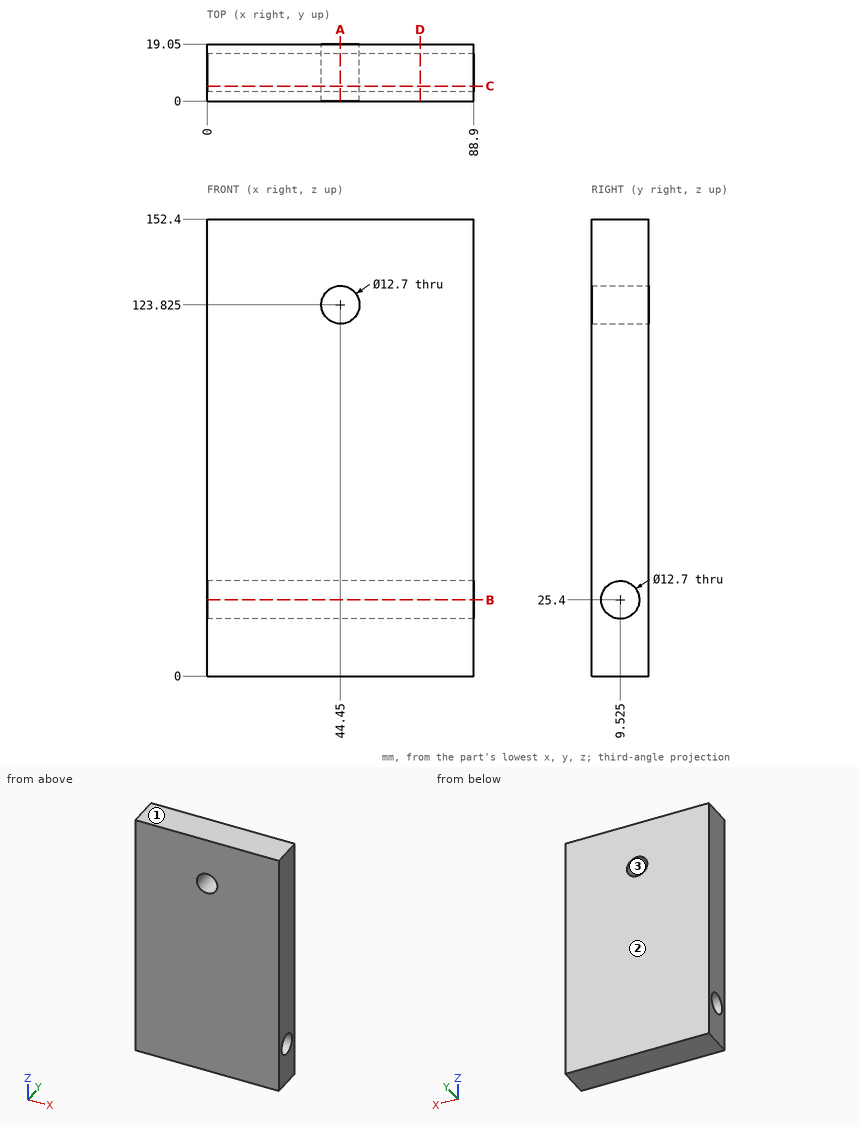
Study the drawing (mm; zero at the part's minimum x, y, z) and answer. Coordinates: 2 decimals unless noted, no trailing zeros. Write each loop counter-clockwise with the first axis right and the second up, starting at its lowest first coordinate (ties: lowest second). Pieces come first, ordered by that corner, then holes. Notation, with made-up numbers: (-15.75, 86.5) - (25.25, 86.5) arc R16 ccw to (25.25, 106.5) - close; hole circle Ø1 at (74.25, 82). An arc over 180 degrees is marked (long way). One line per item, written item: value.
1) Find section B-B (z = 25.4). Give the vertices of the cut face in (x, y) (3 decimals).
Geometry check:
outline: (0, 0) - (88.9, 0) - (88.9, 3.175) - (0, 3.175) - close; (0, 15.875) - (88.9, 15.875) - (88.9, 19.05) - (0, 19.05) - close
2) This flat-tipped pin is pushed along its axis until it touches: pin 1 Ø7.5 at (x, z) = (44.45, 123.825) entering from -Y. Where does it stop, or does it pass through?
Geometry check:
pin 1: passes through
3) Find section C-C (y = 5). Give the vertices of the cut face in (x, z) (3 decimals), and give its area (3 significant figures).
Geometry check:
outline: (0, 0) - (88.9, 0) - (88.9, 20.945) - (0, 20.945) - close; (0, 29.855) - (88.9, 29.855) - (88.9, 152.4) - (0, 152.4) - close; hole circle Ø12.7 at (44.45, 123.825)
area: 12,600 mm2
4) Find section A-A (x = 44.45). Give the vertices of the cut face in (y, z) (3 decimals), and give its area (3 significant figures).
Geometry check:
outline: (0, 0) - (19.05, 0) - (19.05, 117.475) - (0, 117.475) - close; (0, 130.175) - (19.05, 130.175) - (19.05, 152.4) - (0, 152.4) - close; hole circle Ø12.7 at (9.525, 25.4)
area: 2,530 mm2
5) Consider line 1 along Z through (x, y) = (15.5, 9); line 2 along Z through (x, y) = (40, 12.75); line 3 along Z through (x, y) = (43.5, 11.75). Determine where each line is inside the solid, lowest interval first. Write a range as from..to.
Geometry check:
line 1: z = 0..19.07, 31.73..152.4
line 2: z = 0..19.93, 30.87..119.3, 128.35..152.4
line 3: z = 0..19.45, 31.35..117.55, 130.1..152.4
6) For a pull along Z with two mould halves and no side action, classify the marked faces 1, 2 and 3 as pulls with the +Z half, pulls with the -Z half, needs draft (parallel to the pull), parting line crosses it, or undercut.
Geometry check:
face 1: pulls with the +Z half
face 2: needs draft
face 3: undercut
7) Find section D-D (x = 71). Give the vertices of the cut face in (y, z) (3 decimals), and give its area (3 significant figures).
Geometry check:
outline: (0, 0) - (19.05, 0) - (19.05, 152.4) - (0, 152.4) - close; hole circle Ø12.7 at (9.525, 25.4)
area: 2,780 mm2
